Check sheet for the drawn part. Datum: minimum x, y, z corner. Units: mm. Round coordinates to 2 decimals unless told otherwise and drop trailing zeros. Loops run counter-clockwise (first coordinate to the right, second up) from the corner with the lowest first, then second, coordinate; pieces in that order, holes last. Notation, with made-up numbers: (66, 13) - (81, 13) arc R32 ccw to (81, 41) - close; hole circle Ø7 at (24, 28.5). An arc over 180 degrees is marked (long way). Use CSV: the item, a comma, the result in double quotes.
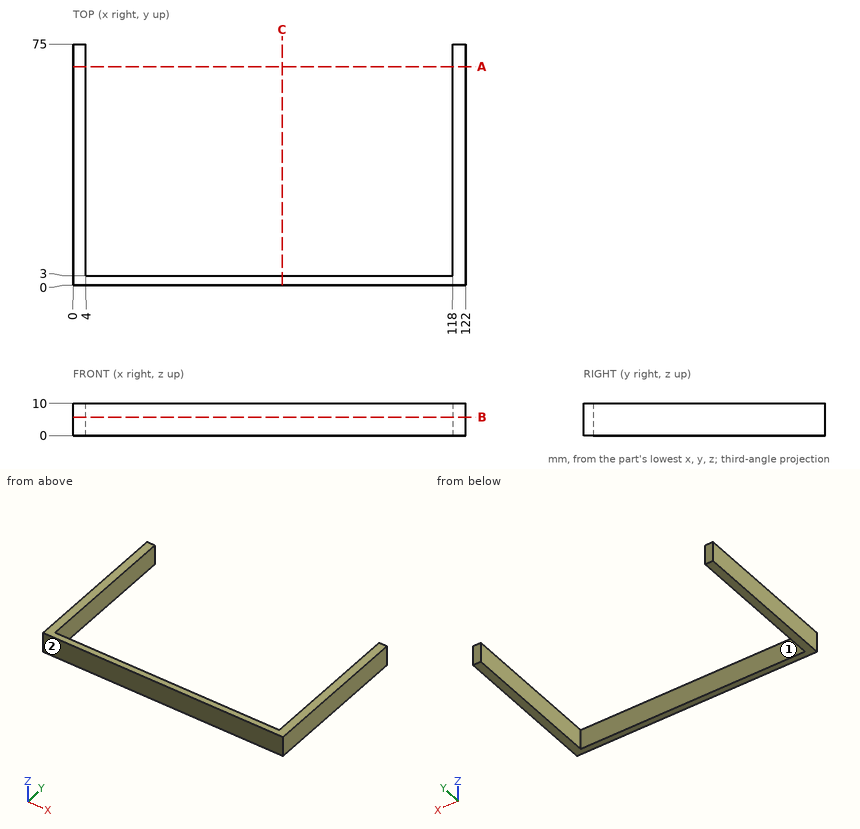
1) Gauge pin test, flat end, axial feed: pin 1 Ø5 at (x, z) = (58, 3) entering from +Y. Record the tip position at first contact, or that the pin passes through.
Returned:
pin 1,"stops at y = 3"
2) Cross-section at B-B, the plane z = 5.75. Record the cut outline in (x, y), then the cut area to 3 significant figures.
Returned:
outline,"(0, 0) - (122, 0) - (122, 75) - (118, 75) - (118, 3) - (4, 3) - (4, 75) - (0, 75) - close"
area,"942 mm²"
3) Mould release check, pull along X, two halves, no side actions. Record for the marked faces 1 and 2: +X half, -X half, draft (parallel to the pull), parting line (faces both ways), or undercut.
Returned:
face 1,"undercut"
face 2,"draft"
4) Thickness scan on probe 1 along X at (y, z) = (27, 3); probe 2 along Y at (x, z) = (40, 2). Record the ranges inside material, lowest first. Write a range as [from, to].
Returned:
probe 1,"x = [0, 4], [118, 122]"
probe 2,"y = [0, 3]"
5) Cross-section at A-A, the plane y = 68. Record the cut outline in (x, z).
Returned:
outline,"(0, 0) - (4, 0) - (4, 10) - (0, 10) - close; (118, 0) - (122, 0) - (122, 10) - (118, 10) - close"
6) Cross-section at C-C, the plane x = 65. Record the cut outline in (y, z), then the cut area to 3 significant figures.
Returned:
outline,"(0, 0) - (3, 0) - (3, 10) - (0, 10) - close"
area,"30.0 mm²"
